```python
from build123d import *

# Parameters (mm, degrees)
F0_W      = 86
F0_H      = 86
F1_DEPTH  = 150
F3_D      = 6.5
F4_R      = 36.5
F5_DEPTH  = 1.6
F7_DEPTH  = 12
F9_DEPTH  = 25
F10_W     = 16.4
F10_H     = 16.4
F10_R     = 3.25
F11_DEPTH = 140


with BuildPart() as f1:
    # F0 (on Top) → F1 (new body)
    with BuildSketch(Plane.XY):
        Rectangle(F0_W, F0_H)
    extrude(amount=F1_DEPTH)

    # F3 (through all)
    with Locations(Plane.XY.offset(150)):
        with Locations((-34.8, 34.8), (34.8, 34.8), (34.8, -34.8), (-34.8, -34.8)):
            Hole(F3_D / 2)

    # F4 (on face) → F5 (join)
    with BuildSketch(Plane.XY.offset(150)):
        Circle(F4_R)
    extrude(amount=F5_DEPTH)

    # F6 (on face) → F7 (join)
    with BuildSketch(Plane.XY.offset(151.6)):
        with BuildLine():
            Line((0, 6), (3.6055512755, 6))
            ThreePointArc((3.6055512755, 6), (0, 7), (-3.6055512755, 6))
            Line((-3.6055512755, 6), (0, 6))
        make_face()
        with BuildLine():
            ThreePointArc((-6, 3.6055512755), (-7, 0), (-6, -3.6055512755))
            Line((-6, -3.6055512755), (-6, 0))
            Line((-6, 0), (-6, 3.6055512755))
        make_face()
        with BuildLine():
            Line((0, 0), (0, -7))
            ThreePointArc((0, -7), (4.9497474683, -4.9497474683), (7, 0))
            Line((7, 0), (0, 0))
        make_face()
        with BuildLine():
            Line((0, 0), (7, 0))
            ThreePointArc((7, 0), (6.0925716626, 3.4468203516), (3.6055512755, 6))
            Line((3.6055512755, 6), (0, 6))
            Line((0, 6), (0, 0))
        make_face()
        with BuildLine():
            ThreePointArc((-6, -3.6055512755), (-3.4468203516, -6.0925716626), (0, -7))
            Line((0, -7), (0, 0))
            Line((0, 0), (-6, 0))
            Line((-6, 0), (-6, -3.6055512755))
        make_face()
        with BuildLine():
            Line((-6, 0), (0, 0))
            Line((0, 0), (0, 6))
            Line((0, 6), (-3.6055512755, 6))
            ThreePointArc((-3.6055512755, 6), (-4.9497474683, 4.9497474683), (-6, 3.6055512755))
            Line((-6, 3.6055512755), (-6, 0))
        make_face()
    extrude(amount=F7_DEPTH)

    # F8 (on face) → F9 (join)
    with BuildSketch(Plane.XY.offset(163.6)):
        with BuildLine():
            ThreePointArc((0, -7), (4.9497474683, -4.9497474683), (7, 0))
            Line((7, 0), (0, 0))
            Line((0, 0), (0, -7))
        make_face()
        with BuildLine():
            Line((0, 0), (7, 0))
            ThreePointArc((7, 0), (6.0925716626, 3.4468203516), (3.6055512755, 6))
            Line((3.6055512755, 6), (0, 6))
            Line((0, 6), (0, 0))
        make_face()
        with BuildLine():
            ThreePointArc((-6, -3.6055512755), (-3.4468203516, -6.0925716626), (0, -7))
            Line((0, -7), (0, 0))
            Line((0, 0), (-6, 0))
            Line((-6, 0), (-6, -3.6055512755))
        make_face()
        with BuildLine():
            Line((-6, 0), (0, 0))
            Line((0, 0), (0, 6))
            Line((0, 6), (-3.6055512755, 6))
            ThreePointArc((-3.6055512755, 6), (-4.9497474683, 4.9497474683), (-6, 3.6055512755))
            Line((-6, 3.6055512755), (-6, 0))
        make_face()
    extrude(amount=F9_DEPTH)

    # F10 (on face) → F11 (cut)
    with BuildSketch(Plane(origin=(0, 0, 0), x_dir=(1, 0, 0), z_dir=(0, 0, -1))):
        with Locations((-34.8, 34.8)):
            Rectangle(F10_W, F10_H)
        with Locations((-34.8, 34.8)):
            Circle(F10_R, mode=Mode.SUBTRACT)
        with Locations((34.8, 34.8)):
            Rectangle(F10_W, F10_H)
        with Locations((34.8, 34.8)):
            Circle(F10_R, mode=Mode.SUBTRACT)
        with Locations((34.8, -34.8)):
            Rectangle(F10_W, F10_H)
        with Locations((34.8, -34.8)):
            Circle(F10_R, mode=Mode.SUBTRACT)
        with Locations((-34.8, -34.8)):
            Rectangle(F10_W, F10_H)
        with Locations((-34.8, -34.8)):
            Circle(F10_R, mode=Mode.SUBTRACT)
    extrude(amount=-F11_DEPTH, mode=Mode.SUBTRACT)


solid = f1.part
```
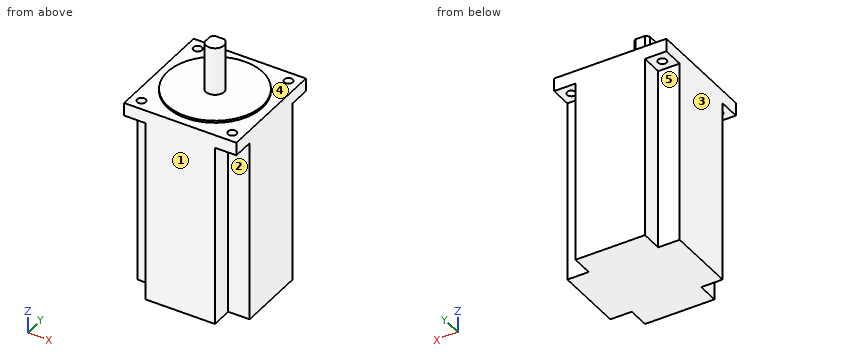
For this review, take the finished solid that the model builds, in its own axes (mm). Face numbers are marked on the shaded views. A direction names the side the tool comes from. Give positions to 0.01 mm unless a question says otherwise; leave off trailing zeros. Write each loop counter-clockwise with the first axis right and the second up, starting at its lowest first coordinate (ties: lowest second). Pieces come first, ordered by that corner, then holes.
Item 1: Take a section at A-A (z = 136.5). Give the boundary of the cut face in (x, y), and give its area (3 significant figures).
Item 2: Insertion check: P1, Ø5, axis at y = -31.5, z = 82.5, coming from the +X side; P2, Ø7.5, axis at x = -34.8, y = -34.8, coming from the -Z side; P3, Ø8, axis at y = 0.5, z = 177.5, coming from the -X side; P4, Ø12, axis at x = 31, z = 163, coming from the -Y side. Each pin has a flat end and moves straight along its axis. Give the tip position at first contact, or say it passes through.
Item 3: Wall thickness on probe 1 along Y at (x, z) = (34.8, 147.5); probe 2 along Y at (x, z) = (-34, 144); probe 3 along Z at (x, y) = (3, 38): over which ranges is each line inside the solid? List them lowest first.
Item 4: Machinability: for the marked faces 1, 2, 3, 4 and 5, which of the approach directions +Z, -Z, +X, -X, +Y, -Y give a long, thin tool a straight path to every point of the face, cutting with its end or side? Answer none if there is none.
Item 5: Take a section at D-D (x = 22.5). Give the boundary of the cut face in (y, z), and give its area (3 significant figures).
Item 6: Take a section at B-B (x = 0). Give the boundary of the cut face in (y, z).
Item 7: Take a section at C-C (y = 0). Give the boundary of the cut face in (x, z).
Established:
1. outline: (-43, -26.6) - (-26.6, -26.6) - (-26.6, -43) - (26.6, -43) - (26.6, -26.6) - (43, -26.6) - (43, 26.6) - (26.6, 26.6) - (26.6, 43) - (-26.6, 43) - (-26.6, 26.6) - (-43, 26.6) - close
1. area: 6,320 mm2
2. P1: stops at x = 26.6
2. P2: stops at z = 140
2. P3: stops at x = -6
2. P4: passes through
3. probe 1: y = -43 to -38.05, -31.55 to 31.55, 38.05 to 43
3. probe 2: y = -43 to -37.95, -31.65 to 31.65, 37.95 to 43
3. probe 3: z = 0 to 150
4. face 1: +Z, -Z, +X, -X, -Y
4. face 2: -Z, +X, -Y
4. face 3: +Z, -Z, -X, +Y, -Y
4. face 4: +Z
4. face 5: -Z, -X, +Y
5. outline: (-43, 0) - (43, 0) - (43, 150) - (28.74, 150) - (28.74, 151.6) - (-28.74, 151.6) - (-28.74, 150) - (-43, 150) - close
5. area: 13,000 mm2
6. outline: (-43, 0) - (43, 0) - (43, 150) - (36.5, 150) - (36.5, 151.6) - (7, 151.6) - (7, 163.6) - (6, 163.6) - (6, 188.6) - (-7, 188.6) - (-7, 151.6) - (-36.5, 151.6) - (-36.5, 150) - (-43, 150) - close
7. outline: (-43, 0) - (43, 0) - (43, 150) - (36.5, 150) - (36.5, 151.6) - (7, 151.6) - (7, 188.6) - (-6, 188.6) - (-6, 163.6) - (-7, 163.6) - (-7, 151.6) - (-36.5, 151.6) - (-36.5, 150) - (-43, 150) - close
